from build123d import *

# Parameters (mm, degrees)
ESQUISSE1_R                  = 1.5
BOSS_EXTRU_1_DEPTH           = 3
ESQUISSE2_W                  = 9
ESQUISSE2_H                  = 9
BOSS_EXTRU_2_DEPTH           = 8
ESQUISSE3_R                  = 1.5
ENL_V_MAT_EXTRU_1_DEPTH      = 32.261930151
ENL_V_MAT_EXTRU_2_DEPTH      = 7
CONG_1_R                     = 5
CONG_2_R                     = 4
CONG_3_R                     = 4
ENL_V_MAT_EXTRU_3_DEPTH      = 44.608458759
ENL_V_MAT_EXTRU_3_DEPTH_BACK = 44.608458759
ESQUISSE5_R                  = 14.5


# Some blends are built 0.0001 mm under size
with BuildPart() as part:
    # Esquisse1 → Boss.-Extru.1 (new body)
    with BuildSketch(Plane(origin=(0, 0, 0), x_dir=(1, 0, 0), z_dir=(0, 1, 0))):
        Polygon((-36.663695412, 22.255522388), (-36.663695412, 13.255522388), (-17.663695412, 13.255522388), (-17.663695412, -11.854477612), (-36.663695412, -11.854477612), (-36.663695412, -20.854477612), (-8.663695412, -20.854477612), (-8.663695412, 22.255522388), align=None)
        with Locations(Location((-32.163695412, 17.755522388, 0), (0, 0, 270))):
            Circle(ESQUISSE1_R, mode=Mode.SUBTRACT)
        with Locations(Location((-11.163695412, 17.755522388, 0), (0, 0, 270))):
            Circle(ESQUISSE1_R, mode=Mode.SUBTRACT)
        with Locations(Location((-32.163695412, -16.354477612, 0), (0, 0, 270))):
            Circle(ESQUISSE1_R, mode=Mode.SUBTRACT)
        with Locations(Location((-11.163695412, -16.354477612, 0), (0, 0, 270))):
            Circle(ESQUISSE1_R, mode=Mode.SUBTRACT)
    extrude(amount=BOSS_EXTRU_1_DEPTH)

    # Esquisse2 → Boss.-Extru.2 (add)
    with BuildSketch(Plane(origin=(0, 3, 0), x_dir=(1, 0, 0), z_dir=(0, 1, 0))):
        with Locations((-13.163695412, 0.700522388)):
            Rectangle(ESQUISSE2_W, ESQUISSE2_H)
    extrude(amount=BOSS_EXTRU_2_DEPTH)

    # Esquisse3 → Enlèv. mat.-Extru.1 (cut, through all)
    with BuildSketch(Plane.ZY.offset(17.663695412)):
        with Locations((-0.700522388, 6.5)):
            Circle(ESQUISSE3_R)
    extrude(amount=-ENL_V_MAT_EXTRU_1_DEPTH, mode=Mode.SUBTRACT)

    # Esquisse4 → Enlèv. mat.-Extru.2 (cut)
    with BuildSketch(Plane.ZY.offset(17.663695412)):
        Polygon((0.786926245, 3.564442716), (2.58546911, 6.320389661), (1.098020477, 9.255946944), (-2.187971021, 9.435557284), (-3.986513886, 6.679610339), (-2.499065254, 3.744053056), align=None)
    extrude(amount=-ENL_V_MAT_EXTRU_2_DEPTH, mode=Mode.SUBTRACT)

    # Congé1
    # the kernel refuses this fillet: 5 mm, written as the material it adds along each edge
    with BuildSketch(Plane(origin=(-17.663695412, 0, 11.854477612), x_dir=(0, 0, -1), z_dir=(0, 1, 0)), Plane(origin=(-17.663695412, 0, -13.255522388), x_dir=(-1, 0, 0), z_dir=(0, 1, 0))) as cong_1_piece_1:
        with BuildLine():
            CenterArc((CONG_1_R, CONG_1_R), CONG_1_R, 180, 90)
            Line((0, CONG_1_R), (0, 0))
            Line((0, 0), (CONG_1_R, 0))
        make_face()
    extrude(amount=3)
    # the kernel refuses this fillet: 5 mm, written as the material it takes off along each edge
    with BuildSketch(Plane(origin=(-8.663695412, -12.5, 20.854477612), x_dir=(0, 0, -1), z_dir=(0, 1, 0)), Plane(origin=(-8.663695412, -12.5, -22.255522388), x_dir=(-1, 0, 0), z_dir=(0, 1, 0)), Plane(origin=(-36.663695412, -12.5, -22.255522388), x_dir=(0, 0, 1), z_dir=(0, 1, 0))) as cong_1_2_piece_1:
        with BuildLine():
            CenterArc((CONG_1_R, CONG_1_R), CONG_1_R, 180, 90)
            Line((0, CONG_1_R), (0, 0))
            Line((0, 0), (CONG_1_R, 0))
        make_face()
    extrude(amount=28, mode=Mode.SUBTRACT)
    with BuildSketch(Plane(origin=(-36.663695412, -12.5, 20.854477612), x_dir=(0, 0, -1), z_dir=(0, 1, 0)), Plane(origin=(-36.663695412, -12.5, 11.854477612), x_dir=(1, 0, 0), z_dir=(0, 1, 0)), Plane(origin=(-36.663695412, -12.5, -13.255522388), x_dir=(0, 0, -1), z_dir=(0, 1, 0))) as cong_1_2_piece_2:
        with BuildLine():
            CenterArc((CONG_1_R, -CONG_1_R), CONG_1_R, 90, 90)
            Line((0, -CONG_1_R), (0, 0))
            Line((0, 0), (CONG_1_R, 0))
        make_face()
    extrude(amount=28, mode=Mode.SUBTRACT)

    # Congé2
    cong_2_edges = [part.edges().sort_by_distance(p)[0] for p in [
        (-13.163695412, 11, 3.799477612),
        (-13.163695412, 11, -5.200522388),
    ]]
    fillet(cong_2_edges, radius=CONG_2_R)

    # Congé3
    cong_3_edges = [part.edges().sort_by_distance(p)[0] for p in [
        (-13.163695412, 3, 3.799477612),
        (-13.163695412, 3, -5.200522388),
    ]]
    fillet(cong_3_edges, radius=CONG_3_R - 0.0001)  # a hair under: the kernel refuses the full size

    # Esquisse5 → Enlèv. mat.-Extru.3 (cut, two sides: drawn at the far end of the back side and taken through both)
    with BuildSketch(Plane(origin=(0, 3, 0), x_dir=(1, 0, 0), z_dir=(0, 1, 0)).offset(-ENL_V_MAT_EXTRU_3_DEPTH_BACK)):
        with Locations((-28.663695412, 0.700522388)):
            Circle(ESQUISSE5_R)
    extrude(amount=ENL_V_MAT_EXTRU_3_DEPTH + ENL_V_MAT_EXTRU_3_DEPTH_BACK, mode=Mode.SUBTRACT)


solid = part.part
Geometry: final body of the model. Coordinates: model frame, mm. A direction names the side the tool comes from. Give positions to 0.01 mm unless a question says otherwise; leave off trailing zeros. Write each loop counter-clockwise with the first axis right and the second up, starting at its lowest first coordinate (ties: lowest second). Pieces come first, ordered by that corner, then holes. Notation, with made-up numbers: (77, 47) -> (129, 47) arc R35 ccw to (129, 84) -> close; hole circle Ø10 at (45, 56). An arc over 180 degrees is marked (long way). Answer as a JSON object with one key per item and string values.
1. Ray query, probe 1 along Y at (x, z) = (-30.25, 16); probe 2 along Z at (x, y) = (-14, 5.5); probe 3 along X at (y, z) = (8.75, -1). Return the intervals inside material, ascending. Write a range as from..to.
Ans:
{"probe 1": "y = 0..3", "probe 2": "z = -5.49..-3.39, 2.05..4.09", "probe 3": "x = -10.66..-8.66"}
2. Cut plane A-A on x = -33. Output: boundary loops of the cut face in (y, z).
Ans:
{"outline": "(0, -22.07) -> (3, -22.07) -> (3, -19) -> (0, -19) -> close; (0, -16.51) -> (3, -16.51) -> (3, -14.54) -> (0, -14.54) -> close; (0, 13.14) -> (3, 13.14) -> (3, 15.11) -> (0, 15.11) -> close; (0, 17.6) -> (3, 17.6) -> (3, 20.67) -> (0, 20.67) -> close"}
3. Access query for faces 1 (the flat face through (-20, 3, -17)), 2 (the flat face through (-10.664, 8, 0)), 3 (the cylindrical face through (-35.9, 1.5, 14.2)), 4 (the cylindrical face through (-27.36, 1.48, -15.14)), 5 (the cylindrical face through (-35.056, 1.479, 19.528)). Directions: +Z, -Z, +X, -X, +Y, -Y. A direction counts if a zero-diameter tool reaches every point of the face in a straight line with its end or side. Return the directions, or none.
Ans:
{"face 1": "-Z, +X, -X, +Y", "face 2": "-X", "face 3": "-X, +Y, -Y", "face 4": "+Y, -Y", "face 5": "+Z, -X, +Y, -Y"}
4. Cut plane D-D on x = -27.5. Output: boundary loops of the cut face in (y, z).
Ans:
{"outline": "(0, -22.26) -> (3, -22.26) -> (3, -15.15) -> (0, -15.15) -> close; (0, 13.75) -> (3, 13.75) -> (3, 20.85) -> (0, 20.85) -> close"}
5. Cut plane B-B on y = 7.5. Output: boundary loops of the cut face in (x, z), and give its area (3 significant figures).
Ans:
{"outline": "(-14.87, -5.17) -> (-8.66, -5.17) -> (-8.66, -1.82) -> (-10.66, -1.82) -> (-10.66, -3.45) -> (-14.43, -3.45) arc R14.5 cw to start; (-14.87, 3.77) arc R14.5 cw to (-14.42, 1.99) -> (-10.66, 1.99) -> (-10.66, 0.42) -> (-8.66, 0.42) -> (-8.66, 3.77) -> close", "area": "27.3 mm^2"}
6. Mould query, pull axis Z, two halves, no side actions, for faces 6 (the cylindrical face through (-10.17, 1.48, 19.43)), 7 (the cylindrical face through (-35.938, 1.479, -15.661)), 8 (the cylindrical face through (-11.728, 9.859, -3.998)). Classes: pulls with the +Z half, pulls with the -Z half, needs draft (parallel to the pull), parting line crosses it, or undercut.
Ans:
{"face 6": "pulls with the +Z half", "face 7": "undercut", "face 8": "pulls with the -Z half"}
7. Cut plane C-C on x = -22.5. Output: boundary loops of the cut face in (y, z), and give its area (3 significant figures).
Ans:
{"outline": "(0, -22.26) -> (3, -22.26) -> (3, -13.83) -> (0, -13.83) -> close; (0, 12.42) -> (3, 12.42) -> (3, 20.85) -> (0, 20.85) -> close", "area": "50.6 mm^2"}
8. Contact query for flat-ended pins moving along their axis: pin 1 (4 mm diameter, centred on x = -28, z = 12, fed in from +Y); pin 2 (1.8 mm diameter, centred on x = -11.16, z = 16.35, fed in from +Y); pin 3 (6 mm diameter, centred on y = 6, z = -2, fed in from -X); pin 4 (1.8 mm diameter, centred on y = 6, z = 0, fed in from -X). Output: stop coordinate, or through.
Ans:
{"pin 1": "stops at y = 3", "pin 2": "passes through", "pin 3": "stops at x = -14.82", "pin 4": "stops at x = -10.66"}
